Verification items for the finished model (mm, model axes). Round coordinates to 2 decimals unless told otherwise and drop trailing zeros. Loops run counter-clockwise (first coordinate to the right, second up) from the corner with the lowest first, then second, coordinate; pieces in that order, holes last.
from build123d import *

# Parameters (mm, degrees)
F0_W     = 76.2
F0_H     = 101.6
F1_DEPTH = 25.4
F2_R     = 24.034722
F3_DEPTH = 50.801
F4_R     = 5.08


with BuildPart() as f1:
    # F0 (on Front) → F1 (new body, symmetric)
    with BuildSketch(Plane.XZ):
        Rectangle(F0_W, F0_H)
    extrude(amount=F1_DEPTH, both=True)

    # F2 (on face) → F3 (cut, through all)
    with BuildSketch(Plane.XZ.offset(25.4)):
        Circle(F2_R)
    extrude(amount=-F3_DEPTH, mode=Mode.SUBTRACT)

    # F4
    f4_edges = [f1.edges().sort_by_distance(p)[0] for p in [
        (-38.1, 0, 50.8),
        (38.1, 0, 50.8),
        (38.1, 0, -50.8),
        (-38.1, 0, -50.8),
    ]]
    fillet(f4_edges, radius=F4_R)


solid = f1.part
1. Section check A-A (z = 0). Enter the section's corners in (x, y), then the cut area to 3 significant figures.
2. Section check C-C (y = 3). Enter the section's corners in (x, z).
3. Section check B-B (x = 0). Enter the section's corners in (y, z).
4. Scan lines: L1, parallel to Z at x = 0, y = 6; L2, parallel to X at y = -6.5, z = 14; L3, parallel to X at y = -5.5, z = -9. Record each from-to range of solid material in increasing order.
5. Release check for a two-part mould opening along X. For faces 1 (the face through (36.572, 0.356, 49.351)), 2 (the face through (-38.1, 0, -1)), 3 (the face through (-24.01, -0.36, 1.06)), 4 (the face through (0, 0, 50.8)) record: released by +X, released by -X, zero draft, split by the parting line, or undercut.
Taken from the geometry:
1. outline: (-38.1, -25.4) - (-24.03, -25.4) - (-24.03, 25.4) - (-38.1, 25.4) - close; (24.03, -25.4) - (38.1, -25.4) - (38.1, 25.4) - (24.03, 25.4) - close
1. area: 1,430 mm2
2. outline: (-38.1, -45.72) arc R5.08 ccw to (-33.02, -50.8) - (33.02, -50.8) arc R5.08 ccw to (38.1, -45.72) - (38.1, 45.72) arc R5.08 ccw to (33.02, 50.8) - (-33.02, 50.8) arc R5.08 ccw to (-38.1, 45.72) - close; hole circle Ø48.07 at (0, 0)
3. outline: (-25.4, -50.8) - (25.4, -50.8) - (25.4, -24.03) - (-25.4, -24.03) - close; (-25.4, 24.03) - (25.4, 24.03) - (25.4, 50.8) - (-25.4, 50.8) - close
4. L1: z = -50.8 to -24.03, 24.03 to 50.8
4. L2: x = -38.1 to -19.54, 19.54 to 38.1
4. L3: x = -38.1 to -22.29, 22.29 to 38.1
5. face 1: released by +X
5. face 2: released by -X
5. face 3: undercut
5. face 4: zero draft
